from build123d import *

# Parameters (mm, degrees)
SKETCH3_W           = 40.386
SKETCH3_H           = 19.558
BOSS_EXTRUDE2_DEPTH = 26.924
SKETCH4_W           = 53.34
SKETCH4_H           = 19.558
BOSS_EXTRUDE3_DEPTH = 1.651
SKETCH5_R           = 2.5019
CUT_EXTRUDE1_DEPTH  = 3.175
SKETCH6_W           = 40.386
SKETCH6_H           = 19.558
BOSS_EXTRUDE4_DEPTH = 7.9375
BOSS_EXTRUDE5_DEPTH = 1.0795
SKETCH8_R           = 6.35
BOSS_EXTRUDE6_DEPTH = 1.5875
SKETCH10_R          = 2.9972
BOSS_EXTRUDE7_DEPTH = 3.175


with BuildPart() as part:
    # Sketch3 → Boss-Extrude2 (new body)
    with BuildSketch(Plane.XY):
        with Locations((-53.574618647, -12.967080077)):
            Rectangle(SKETCH3_W, SKETCH3_H)
    extrude(amount=BOSS_EXTRUDE2_DEPTH)

    # Sketch4 → Boss-Extrude3 (add)
    with BuildSketch(Plane.XY.offset(26.924)):
        with Locations((-53.574618647, -12.967080077)):
            Rectangle(SKETCH4_W, SKETCH4_H)
    extrude(amount=BOSS_EXTRUDE3_DEPTH)

    # Sketch5 → Cut-Extrude1 (cut)
    with BuildSketch(Plane.XY.offset(28.575)):
        with Locations((-77.704618647, -7.887080077)):
            Circle(SKETCH5_R)
        with Locations((-29.444618647, -7.887080077)):
            Circle(SKETCH5_R)
        with Locations((-29.444618647, -18.047080077)):
            Circle(SKETCH5_R)
        with Locations((-77.704618647, -18.047080077)):
            Circle(SKETCH5_R)
    extrude(amount=-CUT_EXTRUDE1_DEPTH, mode=Mode.SUBTRACT)

    # Sketch6 → Boss-Extrude4 (add)
    with BuildSketch(Plane.XY.offset(28.575)):
        with Locations((-53.574618647, -12.967080077)):
            Rectangle(SKETCH6_W, SKETCH6_H)
    extrude(amount=BOSS_EXTRUDE4_DEPTH)

    # Sketch7 → Boss-Extrude5 (add)
    with BuildSketch(Plane.XY.offset(36.5125)):
        with BuildLine():
            Line((-67.036618647, -21.698330077), (-67.036618647, -4.235830077))
            Line((-67.036618647, -4.235830077), (-47.564493582, -4.235830077))
            ThreePointArc((-47.564493582, -4.235830077), (-33.381618647, -12.967080077), (-47.564493582, -21.698330077))
            Line((-47.564493582, -21.698330077), (-67.036618647, -21.698330077))
        make_face()
    extrude(amount=BOSS_EXTRUDE5_DEPTH)

    # Sketch8 → Boss-Extrude6 (add)
    with BuildSketch(Plane.XY.offset(37.592)):
        with Locations((-42.906618647, -13.221080077)):
            Circle(SKETCH8_R)
    extrude(amount=BOSS_EXTRUDE6_DEPTH)

    # Sketch10 → Boss-Extrude7 (add)
    with BuildSketch(Plane.XY.offset(39.1795)):
        with Locations((-42.906618647, -13.221080077)):
            Circle(SKETCH10_R)
    extrude(amount=BOSS_EXTRUDE7_DEPTH)


solid = part.part
The listing builds one solid part. Answer for the finished solid, in the listing's coordinates (mm). A direction names the side the tool comes from. Give positions to 0.01 mm unless a question says otherwise; leave off trailing zeros. Loops run counter-clockwise (first coordinate to the right, second up) from the corner with the lowest first, then second, coordinate; pieces in that order, holes last.
Item 1: A tool of negligible diameter and unlimited length cuts with its end or side. For faces 1 (the flat face through (-30, -13, 26.924)), 2 (the flat face through (-73.768, -13, 13)), 3 (the cylindrical face through (-45.9, -13.1, 40.7)), from which of +Z, -Z, +X, -X, +Y, -Y can it reach the whole face along a straight path? Write none if from no direction.
Derived:
face 1: -Z, +X, +Y, -Y
face 2: -Z, -X, +Y, -Y
face 3: +Z
Item 2: A cutting plane is placed at C-C (x = -39). Give the vertices of the cut face in (y, z) (1 decimal), then the cut area to 3 significant figures.
Derived:
outline: (-22.7, 0) - (-3.2, 0) - (-3.2, 36.5) - (-4.1, 36.5) - (-4.1, 37.6) - (-8.2, 37.6) - (-8.2, 39.2) - (-18.2, 39.2) - (-18.2, 37.6) - (-21.8, 37.6) - (-21.8, 36.5) - (-22.7, 36.5) - close
area: 749 mm2
Item 3: Each of these flat-tipped pins is pushed along its axis until it touches: pin 1 Ø4 at (y, z) = (-9, 9) entering from +X; pin 2 Ø8.5 at (y, z) = (-8.5, 33.5) entering from -X; pin 3 Ø0.5 at (y, z) = (-9.5, 37) entering from -X. Where does it stop, or does it pass through?
Derived:
pin 1: stops at x = -33.38
pin 2: stops at x = -73.77
pin 3: stops at x = -67.04
Item 4: Find the intervals of material crossed by line 1 along X through (y, z) = (-6.25, 28); line 2 along X through (y, z) = (-10.5, 2.5); line 3 along Z through (x, y) = (-44.5, -21), in increasing order.
Derived:
line 1: x = -80.24 to -79.6, -75.81 to -31.34, -27.55 to -26.9
line 2: x = -73.77 to -33.38
line 3: z = 0 to 37.59
Item 5: A cutting plane is placed at A-A (x = -60.5). Give the vertices of the cut face in (y, z), then the cut area to 3 significant figures.
Derived:
outline: (-22.75, 0) - (-3.19, 0) - (-3.19, 36.51) - (-4.24, 36.51) - (-4.24, 37.59) - (-21.7, 37.59) - (-21.7, 36.51) - (-22.75, 36.51) - close
area: 733 mm2
Item 6: Determine the mould class of faces 4 (the cylindrical face through (-27.133, -8.845, 27.761)), 5 (the flat face through (-36, -5, 36.512)), 6 (the cylindrical face through (-27.058, -17.296, 27.761)), 7 (the flat face through (-54, -22.746, 18)) for opening direction Y: +Y half, -Y half, draft (parallel to the pull), parting line (faces both ways), or undercut.
Derived:
face 4: undercut
face 5: draft
face 6: undercut
face 7: -Y half
Item 7: A cutting plane is placed at B-B (z = 20). Give the vertices of the cut face in (x, y).
Derived:
outline: (-73.77, -22.75) - (-33.38, -22.75) - (-33.38, -3.19) - (-73.77, -3.19) - close
